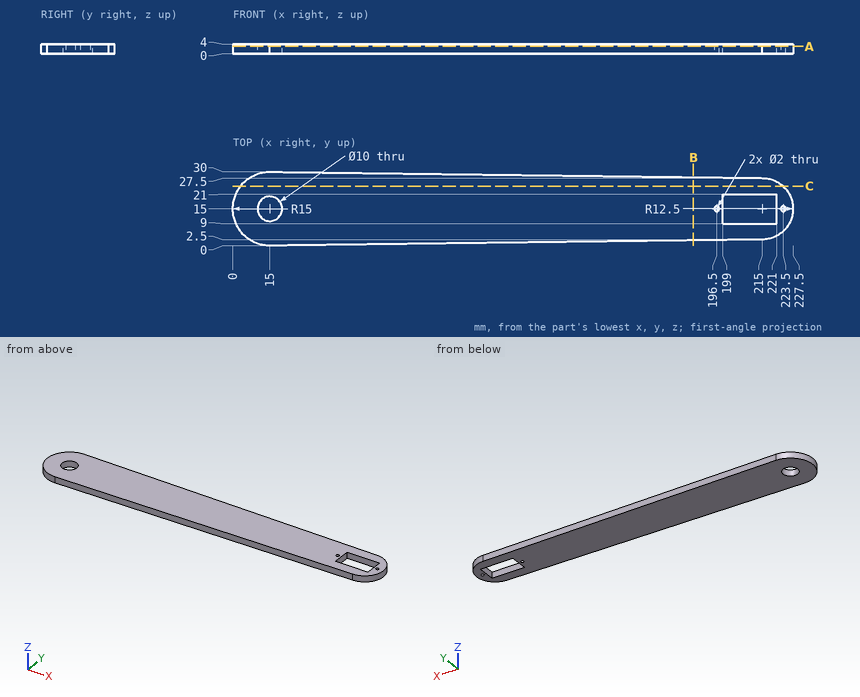
Drawing for the job (mm, zero at the part's lowest x, y, z). Round coordinates to 2 decimals unless told otherwise and drop trailing zeros. Loops run counter-clockwise (first coordinate to the right, second up) from the corner with the lowest first, then second, coordinate; pieces in that order, holes last. Notation, with made-up numbers: (6.5, -36) - (20.5, -36) arc R20 ccw to (20.5, -23) - close; hole circle Ø6 at (7.5, -31). An arc over 180 degrees is marked (long way). Return JSON: item names as keys, results as strings. Group by question number.
Q1. Band-saw the part on C-C on y = 24.25. Give the cut face in (x, z), plus the area to 3 significant figures.
Q2. Band-saw the part on B-B on x = 187. Give the cut face in (y, z).
Q3. Drill centre lines: line 1 along X through (y, z) = (14.75, 2.85); line 2 along X through (y, z) = (13.5, 1.8); line 3 along Y through (x, z) = (15, 2.95). Where is each one in solid material? Low to high. Write a range as [from, to].
Q4. Band-saw the part on A-A on z = 3. Give the cut face in (x, y).
Q5. Flat gauge pins, fed straight in: pin 1 Ø1.2 at (y, z) = (16.5, 3) entering from +X; pin 2 Ø1 at (y, z) = (21.5, 1) entering from -X. Where does each tip first touch, or does it go through?
Solutions:
{
 "1": {"outline": "(3.19, 0) - (223.41, 0) - (223.41, 4) - (3.19, 4) - close", "area": "881 mm^2"},
 "2": {"outline": "(2.15, 0) - (27.85, 0) - (27.85, 4) - (2.15, 4) - close"},
 "3": {"line 1": "x = [0, 10.01], [19.99, 195.53], [197.47, 199], [221, 222.53], [224.47, 227.5]", "line 2": "x = [0.08, 10.23], [19.77, 199], [221, 227.41]", "line 3": "y = [0, 10], [20, 30]"},
 "4": {"outline": "(15, 0) - (215, 2.5) arc R12.5 ccw to (215, 27.5) - (15, 30) arc R15 ccw to start; hole circle Ø10 at (15, 15); hole circle Ø2 at (196.5, 15); hole (199, 9) - (221, 9) - (221, 21) - (199, 21) - close; hole circle Ø2 at (223.5, 15)"},
 "5": {"pin 1": "stops at x = 227.47", "pin 2": "stops at x = 1.25"}
}
